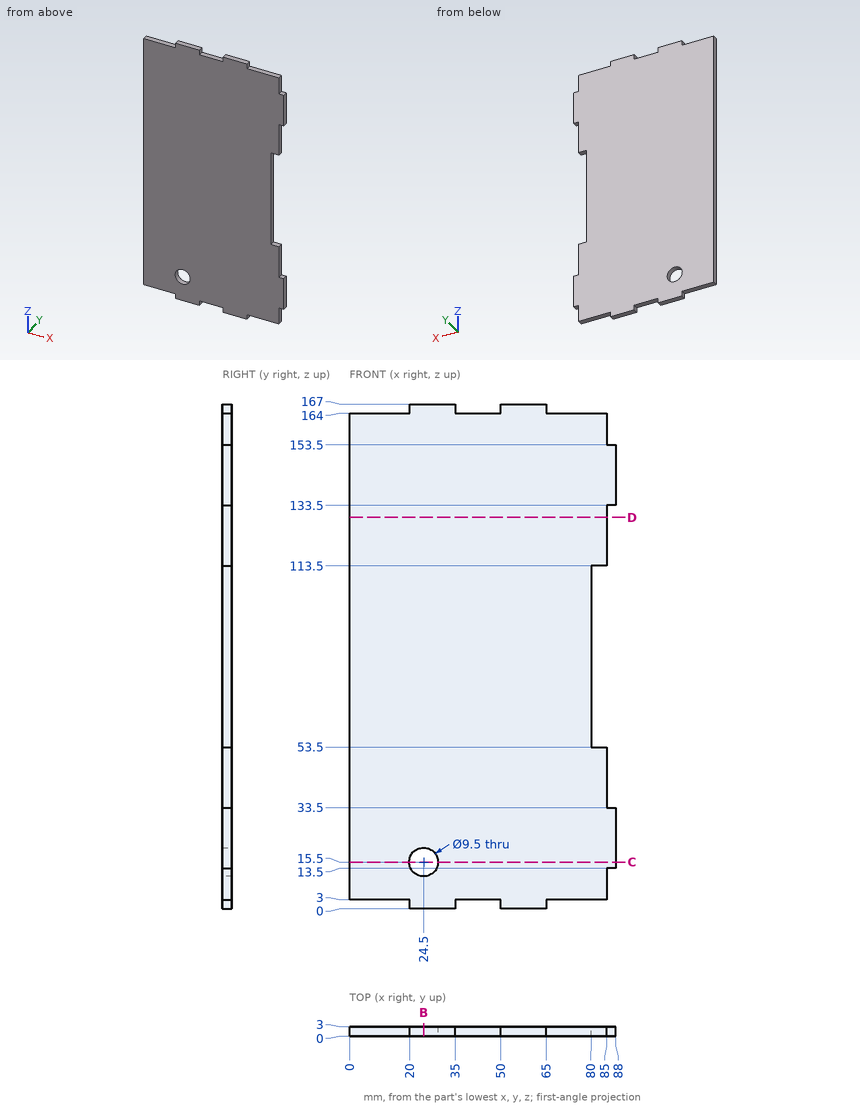
Could you check a few things on this drawing? It's one solid part, dimensions in mm from its lowest x, y, z. Coordinates: 2 decimals unless noted, no trailing zeros. Order: outer loops, then holes, each group sorted by start corner. A loop starts at its lowest first (then second) coordinate and runs counter-clockwise, first axis right, second up. Notation, with made-up numbers: M 40,44.25 L 62,44.25 A22 ccw 62,52.25 Z; hole C -28,-17 d2. An arc over 180 degrees is marked long. Answer as a JSON object with one key per item and string values. Group by question number.
(1) Suppose I cut it at C-C, the plane z = 15.5. Please give me the cut outline in (x, y), then the cut area to 4 significant figures.
(2) Suppose I cut it at D-D, the plane z = 129.5. Please give me the cut outline in (x, y), then the cut area to 3 significant figures.
(3) I need wall thicknesses on probe 1 along X at (y, z) = (0.7, 15.5); probe 2 along X at (y, z) = (0.7, 60.5); probe 3 along Z at (x, y) = (68, 0.2). Which ranges of each line are inside material? Lowest first, please.
(4) Suppose I cut it at B-B, the plane x = 24.5. Please give me the cut outline in (y, z), then the cut area to 4 significant figures.
(5) For pin 1 (0.9 mm diameter, centred on y = 1, z = 165, fed in from -X); pin 2 (0.9 mm diameter, centred on y = 1, z = 48, fed in from +X); pin 3 (1.5 mm diameter, centred on x = 87, y = 1, fed in from +Z); pin 4 (8 mm diameter, centred on x = 62.5, z = 66, fed in from -Y), each with a flat end and sliding along its axis, tell me the tip position at first contact or that it passes through.
Values found:
{
 "1": {"outline": "M 0,0 L 19.75,0 L 19.75,3 L 0,3 Z; M 29.25,0 L 88,0 L 88,3 L 29.25,3 Z", "area": "235.5 mm^2"},
 "2": {"outline": "M 0,0 L 85,0 L 85,3 L 0,3 Z", "area": "255 mm^2"},
 "3": {"probe 1": "x = 0 to 19.75, 29.25 to 88", "probe 2": "x = 0 to 80", "probe 3": "z = 3 to 164"},
 "4": {"outline": "M 0,0 L 3,0 L 3,10.75 L 0,10.75 Z; M 0,20.25 L 3,20.25 L 3,167 L 0,167 Z", "area": "472.5 mm^2"},
 "5": {"pin 1": "stops at x = 20", "pin 2": "stops at x = 85", "pin 3": "stops at z = 153.5", "pin 4": "stops at y = 0"}
}
